Build history of the part. All positions in model axes, mm. A direction names the side the tool comes from. Round coordinates to 2 decimals unless told otherwise and drop trailing zeros. Loops run counter-clockwise (first coordinate to the right, second up) from the corner with the lowest first, then second, coordinate; pieces in that order, holes last. Notation, with made-up numbers: (-28, 56) - (-12, 56) arc R33 cw to (-12, 95) - close; hole circle Ø1 at (32, -14). An arc over 180 degrees is marked (long way). Use a Markdown table: item, result.
from build123d import *

# Parameters (mm, degrees)
FILLET_1_R  = 0.2
HEX_2_DEPTH = 1.56


with BuildPart() as part:
    # Эскиз1 → Body (revolve)
    with BuildSketch(Plane.XY):
        with BuildLine():
            Line((0, 2.375), (0, 0))
            Line((0, 0), (52.75, 0))
            Line((52.75, 0), (52.75, 2.055))
            Line((52.75, 2.055), (52.305, 2.5))
            Line((52.305, 2.5), (2.75, 2.5))
            Line((2.75, 2.5), (2.75, 4.75))
            Line((2.75, 4.75), (2.370164642, 4.75))
            ThreePointArc((2.370164642, 4.75), (0.992749859, 3.754440885), (0, 2.375))
        make_face()
    revolve(axis=Axis((-3.643489966, 0, 0), (-1, 0, 0)))

    # Скругление1
    fillet_1_edges = [part.edges().sort_by_distance(p)[0] for p in [
        (2.75, -2.5, 0),
    ]]
    fillet(fillet_1_edges, radius=FILLET_1_R)

    # Эскиз2 → Вырез-Повернуть1 (revolve, cut)
    with BuildSketch(Plane.XY):
        Polygon((0, 0), (0, 1.5), (1.56, 1.5), (2.426025404, 0), align=None)
    revolve(axis=Axis((2.426025404, 0, 0), (-1, 0, 0)), mode=Mode.SUBTRACT)

    # Эскиз3 → Hex 2 (cut)
    with BuildSketch(Plane.ZY):
        Polygon((-1.5, -0.866025404), (0, -1.732050808), (1.5, -0.866025404), (1.5, 0.866025404), (0, 1.732050808), (-1.5, 0.866025404), align=None)
    extrude(amount=-HEX_2_DEPTH, mode=Mode.SUBTRACT)


solid = part.part
Q1. Drop flat-ended pins along their axis: pin 1 (2 mm diameter, centred on x = 40.5, y = 0, fed in from -Z); pin 2 (2 mm diameter, centred on x = 17.5, y = 2, fed in from +Z); pin 3 (0.6 mm diameter, centred on y = -1, z = 1, fed in from -X); pin 4 (1.7 mm diameter, centred on x = 1, y = -0.5, fed in from +Z). Give the stop position or say it passes through.
Results found:
| item | result |
|---|---|
| pin 1 | stops at z = -2.5 |
| pin 2 | stops at z = 2.29 |
| pin 3 | stops at x = 0 |
| pin 4 | stops at z = 4.43 |
Q2. Cut at B-B, the plane y = 3.75. List the corners of the cut face in (x, z).
Results found:
| item | result |
|---|---|
| outline | (2.37, -2.92) - (2.75, -2.92) - (2.75, 2.92) - (2.37, 2.92) arc R3.77 ccw to start |
Q3. Which spindle directions (+Z, -Z, +X, -X, +Y, -Y) get a long thin tool onto all of the face, cutting with end or side? Do faces 4 (the face through (2.557, 2.192, 4.214)), 5 (the face through (1, 0, 1.5)). Say none if no direction does.
Results found:
| item | result |
|---|---|
| face 4 | +X, -X |
| face 5 | -X |
Q4. Probe line 1 (Y direction, x = 17.5, z = 0); line 2 (Z direction, x = 24, y = 0.5); line 3 (X direction, y = -3.75, z = 1). List the from-to ranges inside material, lowest first.
Results found:
| item | result |
|---|---|
| line 1 | y = -2.5 to 2.5 |
| line 2 | z = -2.45 to 2.45 |
| line 3 | x = 1.12 to 2.75 |
Q5. Pull direction Y, two halves, no side cores. Call faces 1 (the face through (2.75, -2.04, 2.04)), 2 (the face through (27.28, -0.54, 2.44)), 3 (the face through (0.769, -1.305, 0.74)): pulls with the +Y half, pulls with the -Y half, needs draft (parallel to the pull), parting line crosses it, or undercut.
Results found:
| item | result |
|---|---|
| face 1 | needs draft |
| face 2 | parting line crosses it |
| face 3 | undercut |
Q6. Cut at A-A, the plane x = 4.5. List the corners of the cut face in (y, z), plus the area to 3 significant figures.
Results found:
| item | result |
|---|---|
| outline | circle Ø5 at (0, 0) |
| area | 19.6 mm2 |
